Print and shaded views of the part. All mm, measured from the part's lowest x, y and z. A direction names the side the tool comes from. Round coordinates to 2 decimals unless told otherwise and drop trailing zeros. Write each loop counter-clockwise with the first axis right and the second up, starting at its lowest first coordinate (ties: lowest second). Pieces come first, ordered by that corner, then holes. Notation, with made-up numbers: M 9,54.25 L 44,54.25 A13 ccw 44,59.25 Z; hole C 52,37 d3. An arc over 180 degrees is marked long. Write item = value, one per line.
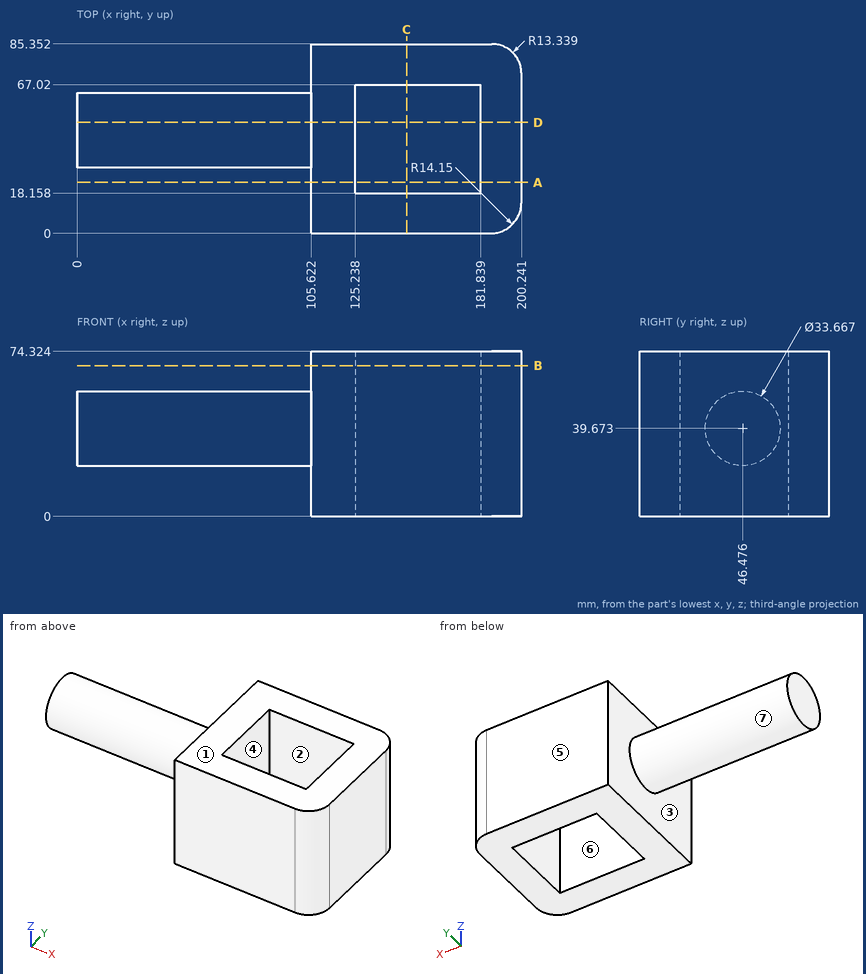
1. Probe probe 1 along Y at (x, z) = (144, 67); probe 2 along X at (y, z) = (49.5, 19); probe 3 along Y at (x, z) = (186.5, 19.5) (1 decimal). List the from-to ranges inside material, lowest first.
Responses:
probe_1 = 0 to 18.16, 67.02 to 85.35
probe_2 = 105.62 to 125.24, 181.84 to 200.24
probe_3 = 0 to 85.4
2. Band-saw the part on D-D (y = 50). List the corners of the cut face in (x, z) (1 decimal), plus the area to 3 significant figures.
Responses:
outline = M 0,23.2 L 105.6,23.2 L 105.6,0 L 125.2,0 L 125.2,74.3 L 105.6,74.3 L 105.6,56.1 L 0,56.1 Z; M 181.8,0 L 200.2,0 L 200.2,74.3 L 181.8,74.3 Z
area = 6,300 mm²
3. Mould opens along X. For the marked faces 1, 2, 3 and 4 say: pulls with the +X half, pulls with the -X half, needs draft (parallel to the pull), parting line crosses it, or undercut.
Responses:
face_1 = needs draft
face_2 = undercut
face_3 = pulls with the -X half
face_4 = undercut
4. Band-saw the part on A-A (y = 23). List the corners of the cut face in (x, z) (1 decimal), plus the area to 3 significant figures.
Responses:
outline = M 105.6,0 L 125.2,0 L 125.2,74.3 L 105.6,74.3 Z; M 181.8,0 L 200.2,0 L 200.2,74.3 L 181.8,74.3 Z
area = 2,830 mm²
5. Band-saw the part on C-C (x = 148.5). List the corners of the cut face in (y, z) (1 decimal), plus the area to 3 significant figures.
Responses:
outline = M 0,0 L 18.2,0 L 18.2,74.3 L 0,74.3 Z; M 67,0 L 85.4,0 L 85.4,74.3 L 67,74.3 Z
area = 2,710 mm²
6. Flat gauge pins, fed straight in: pin 1 (3 mm diameter, centred on y = 31, z = 54, fed in from -X); pin 2 (12 mm diameter, centred on x = 24, y = 66, fed in from +Z) (1 decimal). Where does each tip first touch, or does it go through?
Responses:
pin_1 = 105.62
pin_2 = 49.7
7. Band-saw the part on B-B (z = 68). List the corners of the cut face in (x, y).
Responses:
outline = M 105.62,0 L 186.09,0 A14.15 ccw 200.24,14.15 L 200.24,72.01 A13.34 ccw 186.9,85.35 L 105.62,85.35 Z; hole M 125.24,18.16 L 181.84,18.16 L 181.84,67.02 L 125.24,67.02 Z
8. Tool access for the marked faces 5, 6 and 7: list every direction of +Z, -Z, +X, -X, +Y, -Y with a clear straight run to the whole face (end or side of a thin tool).
Responses:
face_5 = +Z, -Z, +X, -X, +Y
face_6 = +Z, -Z
face_7 = -X
